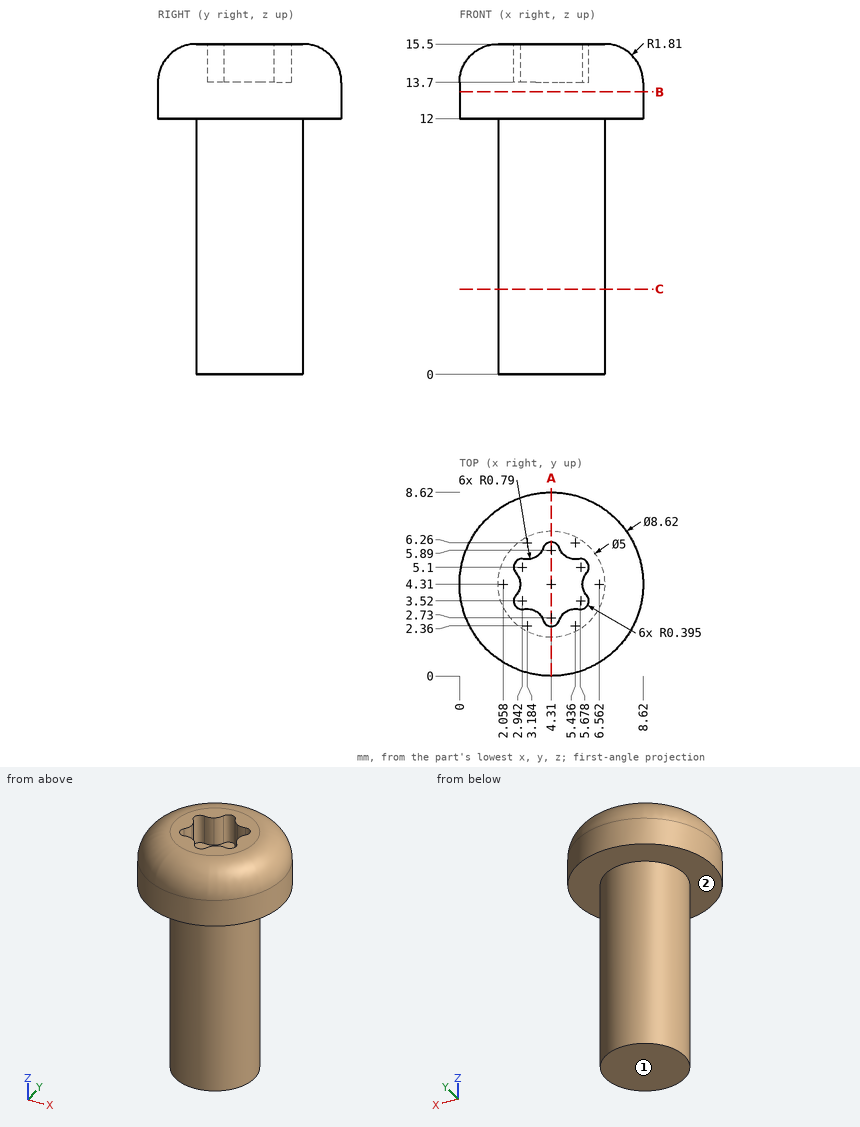
Geometry check sheet. Reference: drawing and pictorial views, mm from the part's lowest x, y, z. A direction names the side the tool comes from. Round coordinates to 2 decimals unless told otherwise and drop trailing zeros. Write each loop counter-clockwise with the first axis right and the second up, starting at its lowest first coordinate (ties: lowest second). Pieces come first, ordered by that corner, then holes. Notation, with made-up numbers: (65.25, 71) -> (119.25, 71) arc R8 ccw to (119.25, 86) -> close; hole circle Ø7 at (26.5, 0.25). An arc over 180 degrees is marked (long way). One line per question, with ' | ' between items. Start each with the question number.
1. Sectioned sample at C-C, the plane z = 4. Record the cut outline in (x, y).
2. Depth check by flat-ended pin: pin 1 (2 mm diameter, centred on x = 3, z = 2.5, fed in from +Y); pin 2 (1 mm diameter, centred on x = 3.5, y = 2, fed in from -Z); pin 3 (3 mm diameter, centred on y = 2.5, z = 9, fed in from +X); pin 4 (1 mm diameter, centred on y = 6, z = 2, fed in from -X). Enter the tip coordinate at first touch or a pass-through.
3. Sectioned sample at B-B, the plane z = 13.25. Record the cut outline in (x, y).
4. Set-up check for the marked faces 1 and 2: record each of +Z, -Z, +X, -X, +Y, -Y from which the full face is reachable in a straight line by a thin tool's end or side.
5. Scan lines: line 1 along X through (y, z) = (4.25, 10.75); line 2 along Z through (x, y) = (3, 4); line 3 along Z through (x, y) = (6.5, 3). Record each from-to range of solid material in increasing order. Write a range as from..to.
6. Sectioned sample at A-A, the plane x = 4.31. Record the cut outline in (y, z) (1 decimal).
Taken from the geometry:
1) outline: circle Ø5 at (4.31, 4.31)
2) pin 1: stops at y = 6.79 | pin 2: stops at z = 0 | pin 3: stops at x = 6.79 | pin 4: stops at x = 2.11
3) outline: circle Ø8.62 at (4.31, 4.31)
4) face 1: -Z, +X, -X, +Y, -Y | face 2: -Z
5) line 1: x = 1.81..6.81 | line 2: z = 0..13.7 | line 3: z = 12..15.5
6) outline: (0, 12) -> (1.8, 12) -> (1.8, 0) -> (6.8, 0) -> (6.8, 12) -> (8.6, 12) -> (8.6, 13.7) arc R1.8 ccw to (6.8, 15.5) -> (6.3, 15.5) -> (6.3, 13.7) -> (2.3, 13.7) -> (2.3, 15.5) -> (1.8, 15.5) arc R1.8 ccw to (0, 13.7) -> close
